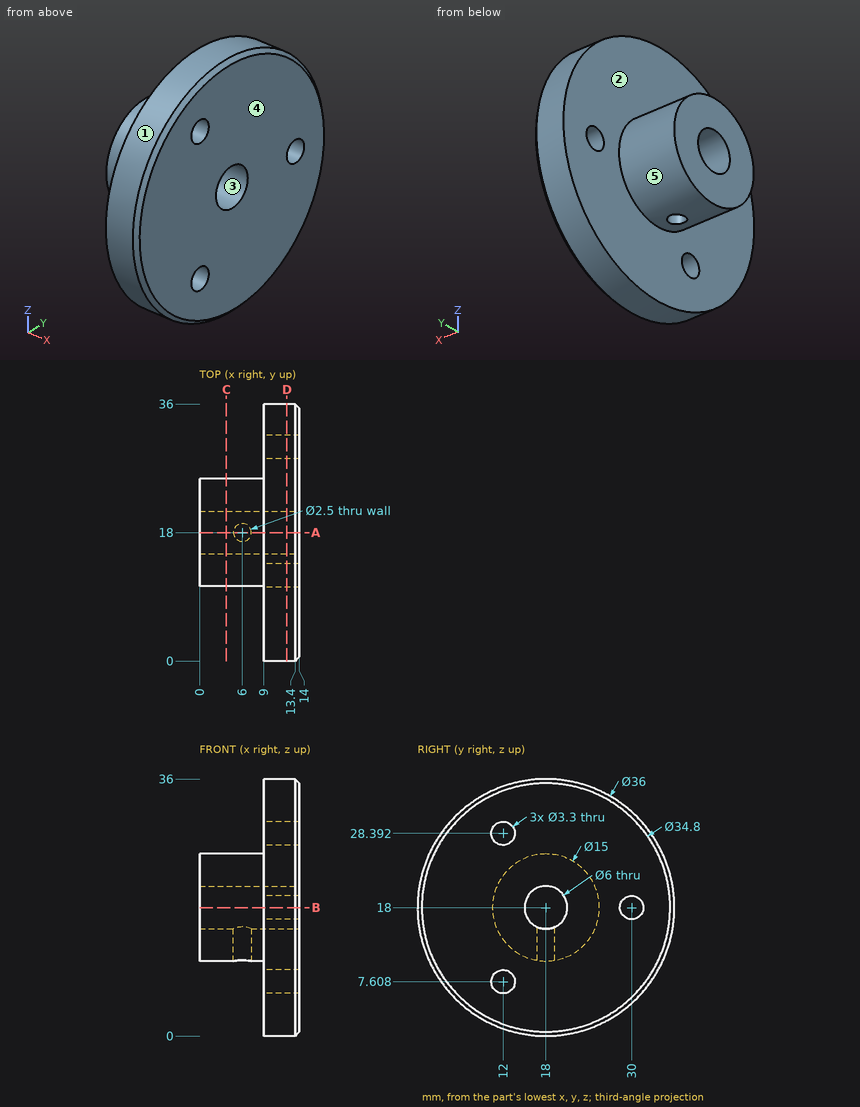
Source: three-view drawing plus pictorial views. Frame: mm from the lowest corner of the part. A direction names the side the tool comes from. Round coordinates to 2 decimals unless told otherwise and drop trailing zeros. Write each loop counter-clockwise with the first axis right and the second up, starting at its lowest first coordinate (ties: lowest second). Pieces come first, ordered by that corner, then holes. Notation, with made-up numbers: M -4.75,52.5 L 52.25,52.5 A11 ccw 52.25,71.5 Z; hole C 43,22 d6. An arc over 180 degrees is marked long. Write each question's results on one line, items separated by ' | '.
Q1. Draft query along Y for the marked faces 1, 2 and 3. Return one class per face: released by +Y, released by -Y, zero draft, split by the parting line, or undercut.
Results:
face 1: split by the parting line | face 2: zero draft | face 3: undercut
Q2. Section query B-B (z = 18). Return loops of the section in (x, y).
Results:
outline: M 0,10.5 L 9,10.5 L 9,0 L 13.4,0 L 14,0.6 L 14,15 L 0,15 Z; M 0,21 L 14,21 L 14,28.35 L 9,28.35 L 9,25.5 L 0,25.5 Z; M 9,31.65 L 14,31.65 L 14,35.4 L 13.4,36 L 9,36 Z
Q3. Section query A-A (y = 18). Return loops of the section in (x, z), and give its area (3 significant figures).
Results:
outline: M 0,10.5 L 4.75,10.5 L 4.75,15 L 0,15 Z; M 0,21 L 14,21 L 14,35.4 L 13.4,36 L 9,36 L 9,25.5 L 0,25.5 Z; M 7.25,10.5 L 9,10.5 L 9,0 L 13.4,0 L 14,0.6 L 14,15 L 7.25,15 Z | area: 219 mm^2
Q4. Section query C-C (x = 3.75). Return loops of the section in (y, z), and give its area (3 significant figures).
Results:
outline: C 18,18 d15; hole C 18,18 d6 | area: 148 mm^2
Q5. Section query D-D (x = 12.25). Return loops of the section in (y, z).
Results:
outline: C 18,18 d36; hole C 12,7.61 d3.3; hole C 12,28.39 d3.3; hole C 18,18 d6; hole C 30,18 d3.3
Q6. Line query: line 1 along Y through (x, z) = (11.75, 18); line 2 along Z through (x, y) = (7.75, 18); line 3 along Y through (x, z) = (4, 16) (1 decimal). Output: solid intervals per line, ascending.
Results:
line 1: y = 0 to 15, 21 to 28.35, 31.65 to 36 | line 2: z = 10.5 to 15, 21 to 25.5 | line 3: y = 10.8 to 15.8, 20.2 to 25.2
Q7. Access query for the marked faces 4 and 5. Directions: +Z, -Z, +X, -X, +Y, -Y. A direction counts if a zero-diameter tool reaches every point of the face in a straight line with its end or side. Return the directions, or none.
Results:
face 4: +Z, -Z, +X, +Y, -Y | face 5: -X
Q8. Pin query (flat end, axial travel): P1, Ø8, axis at x = 3, y = 4.5, coming from the -Z side; P2, Ø3, axis at x = 8.5, z = 4, coming from the -Y side; P3, Ø2, axis at x = 8.5, y = 24, coming from the +Z side; P4, Ø1.5, axis at x = 3.5, y = 17.5, coming from the +Z side. Return the tip coordinate at first contact, or that it passes through.
Results:
P1: passes through | P2: stops at y = 5.13 | P3: stops at z = 35.25 | P4: stops at z = 25.5
